The listing builds one solid part. Answer for the finished solid, in the listing's coordinates (mm). Coordinates: 2 decimals unless noted, no trailing zeros. Write each loop counter-clockwise with the first axis right and the second up, starting at its lowest first coordinate (ties: lowest second). Pieces come first, ordered by that corner, then holes. Notation, with made-up numbers: M -36,1.25 L -19,1.25 A22 ccw -19,14.25 Z; hole C -25.75,-8 d8. An arc over 180 degrees is marked long. Answer as CSV lines item,"result". Start each with the question number.
```python
from build123d import *

# Parameters (mm, degrees)
SKETCH006_R   = 43
SKETCH006_R_2 = 1.5
SKETCH006_R_3 = 9
PAD_DEPTH     = 3.5
CHAMFER_SIZE  = 1.4


with BuildPart() as part:
    # Sketch006 → Pad (new body)
    with BuildSketch(Plane.XY.offset(22)):
        Circle(SKETCH006_R)
        with Locations((0, 36)):
            Circle(SKETCH006_R_2, mode=Mode.SUBTRACT)
        with Locations((31.176915, -18)):
            Circle(SKETCH006_R_2, mode=Mode.SUBTRACT)
        with Locations((-31.176915, -18)):
            Circle(SKETCH006_R_2, mode=Mode.SUBTRACT)
        Circle(SKETCH006_R_3, mode=Mode.SUBTRACT)
    extrude(amount=PAD_DEPTH)

    # Chamfer
    chamfer_edges = [part.edges().sort_by_distance(p)[0] for p in [
        (-32.676915, -18, 22),
        (-1.5, 36, 22),
        (29.676915, -18, 22),
    ]]
    chamfer(chamfer_edges, length=CHAMFER_SIZE)


solid = part.part
```
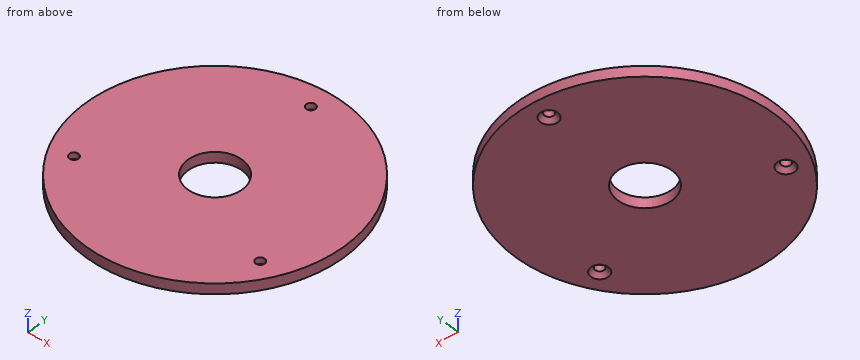
1) Each of these flat-tipped pins is pushed along its axis until it touches: P1, Ø1, axis at x = -14, z = 24, coming from the -Y side; P2, Ø2, axis at x = 33, z = 23.5, coming from the -Y side. Where does it stop, or does it pass through?
2) The part is cut by section A-A (x = -5). Determine the outline of the cut face in (y, z), then the cut area to 3 significant figures.
3) The part is cut by section C-C (z = 24.85). Determine the outline of the cut face in (x, y).
4) Find the intervals of material crossed by line 1 (Y direction, x = 0, z = 24.4); line 2 (Y direction, x = 0, z = 23.25); line 3 (Y direction, x = -32, z = 23.05), in increasing order. Write a range as from..to.
5) The part is cut by section B-B (y = 0). Determine the outline of the cut face in (x, z), then the cut area to 3 significant figures.
6) The part is cut by section D-D (y = -18). Determine the outline of the cut face in (x, z).
Completed:
1,P1,"y = -40.83"
1,P2,"y = -28.72"
2,outline,"M -42.71,22 L -7.48,22 L -7.48,25.5 L -42.71,25.5 Z; M 7.48,22 L 42.71,22 L 42.71,25.5 L 7.48,25.5 Z"
2,area,"247 mm²"
3,outline,"C 0,0 d86; hole C -31.18,-18 d3; hole C 0,0 d18; hole C 0,36 d3; hole C 31.18,-18 d3"
4,line 1,"-43..-9, 9..34.5, 37.5..43"
4,line 2,"-43..-9, 9..34.35, 37.65..43"
4,line 3,"-28.72..-19.66, -16.34..28.72"
5,outline,"M -43,22 L -9,22 L -9,25.5 L -43,25.5 Z; M 9,22 L 43,22 L 43,25.5 L 9,25.5 Z"
5,area,"238 mm²"
6,outline,"M -39.05,22 L -34.08,22 L -32.68,23.4 L -32.68,25.5 L -39.05,25.5 Z; M -29.68,23.4 L -28.28,22 L 28.28,22 L 29.68,23.4 L 29.68,25.5 L -29.68,25.5 Z; M 32.68,23.4 L 34.08,22 L 39.05,22 L 39.05,25.5 L 32.68,25.5 Z"
